Build history of the part. All positions in model axes, mm. Face numbers are marked on the shaded views. A direction names the side the tool comes from. Give positions to 0.01 mm unless a question says otherwise; leave off trailing zeros. Loops run counter-clockwise (first coordinate to the right, second up) from the corner with the lowest first, then second, coordinate; pieces in that order, holes last. Notation, with made-up numbers: (7.5, -12.5) -> (47.5, -12.5) arc R19 cw to (47.5, 6.5) -> close; hole circle Ø5 at (73.5, 86.5). An arc over 180 degrees is marked (long way). Answer as a JSON object with one key per item and string values. Group by question number.
Q1. Two-plate mould, pull along Y, no slides. Class the marked faces 3 and 4: pulls with the +Y half, pulls with the -Y half, needs draft (parallel to the pull), parting line crosses it, or undercut.
Q2. Band-saw the part on B-B, the plane y = 55.5. Write the cut outline in (x, z).
Q3. Drop flat-ended pins along their axis: pin 1 (4 mm diameter, centred on y = 151, z = 32.5, fed in from -X); pin 2 (3 mm diameter, centred on x = 140.5, z = 36.5, fed in from +Y); pin 3 (5 mm diameter, centred on x = 150, z = 96, fed in from +Y). Give the stop position or say it passes through.
Q4. Band-saw the part on A-A, the plane z = 17. Write the cut outline in (x, y), plus the area to 3 significant figures.
Q5. Tool access for the marked faces 1 and 2: list every direction of +Z, -Z, +X, -X, +Y, -Y with a clear straight run to the whole face (end or side of a thin tool).
Q6. Band-saw the part on C-C, the plane x = 102. Write the cut outline in (y, z).
Q7. Wall check: probe 1 along Y at (x, z) = (24.5, 78); probe 2 along Y at (x, z) = (134, 7); probe 3 along Z at (x, y) = (150, 1.5). Give the ranges that are in metal, low to high. Write a range as from..to.
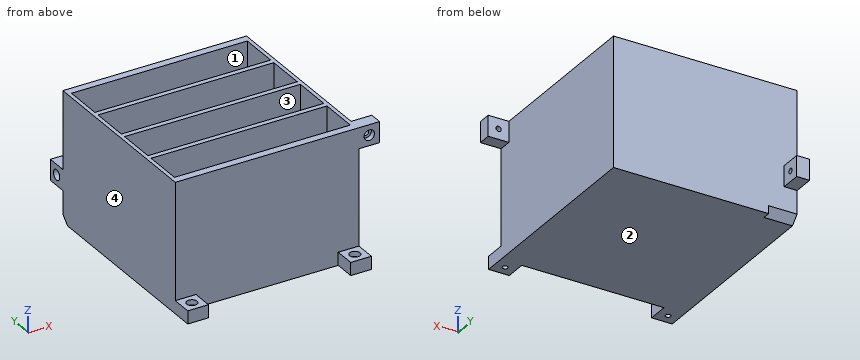
from build123d import *

# Parameters (mm, degrees)
SKETCH_W        = 142
SKETCH_H        = 144
PAD_DEPTH       = 100
SKETCH001_W     = 136
SKETCH001_H     = 30
POCKET_DEPTH    = 95
SKETCH002_W     = 10
SKETCH002_H     = 16
PAD001_DEPTH    = 16
SKETCH003_R     = 4
POCKET001_DEPTH = 4
SKETCH004_R     = 2
POCKET002_DEPTH = 6
SKETCH005_W     = 16
SKETCH005_H     = 10
PAD002_DEPTH    = 16
SKETCH006_R     = 4
POCKET003_DEPTH = 4
SKETCH007_R     = 2
POCKET004_DEPTH = 6
POCKET005_DEPTH = 22
SKETCH009_W     = 10
SKETCH009_H     = 16
PAD003_DEPTH    = 16
SKETCH010_R     = 4
POCKET006_DEPTH = 4
SKETCH011_R     = 2
POCKET007_DEPTH = 6


with BuildPart() as part:
    # Sketch → Pad (new body)
    with BuildSketch(Plane.XY):
        with Locations((71, 72)):
            Rectangle(SKETCH_W, SKETCH_H)
    extrude(amount=PAD_DEPTH)

    # Sketch001 (on Face6 of Pad) → Pocket (cut)
    with BuildSketch(Plane.XY.offset(100)):
        with Locations((71, 123)):
            Rectangle(SKETCH001_W, SKETCH001_H)
        with Locations((71, 89)):
            Rectangle(SKETCH001_W, SKETCH001_H)
        with Locations((71, 55)):
            Rectangle(SKETCH001_W, SKETCH001_H)
        with Locations((71, 21)):
            Rectangle(SKETCH001_W, SKETCH001_H)
    extrude(amount=-POCKET_DEPTH, mode=Mode.SUBTRACT)

    # Sketch002 (on Face1 of Pocket) → Pad001 (join)
    with BuildSketch(Plane(origin=(0, 144, 0), x_dir=(-1, 0, 0), z_dir=(0, 1, 0))):
        with Locations((-5, 32)):
            Rectangle(SKETCH002_W, SKETCH002_H)
    extrude(amount=PAD001_DEPTH)

    # Sketch003 (on Face10 of Pad001) → Pocket001 (cut)
    with BuildSketch(Plane(origin=(0, 0, 0), x_dir=(0, -1, 0), z_dir=(-1, 0, 0))):
        with Locations((-152, 32)):
            Circle(SKETCH003_R)
    extrude(amount=-POCKET001_DEPTH, mode=Mode.SUBTRACT)

    # Sketch004 (on Face33 of Pocket001) → Pocket002 (cut)
    with BuildSketch(Plane(origin=(4, 0, 0), x_dir=(0, -1, 0), z_dir=(-1, 0, 0))):
        with Locations((-152, 32)):
            Circle(SKETCH004_R)
    extrude(amount=-POCKET002_DEPTH, mode=Mode.SUBTRACT)

    # Sketch005 (on Face4 of Pocket002) → Pad002 (join)
    with BuildSketch(Plane.XZ):
        with Locations((8, 5)):
            Rectangle(SKETCH005_W, SKETCH005_H)
        with Locations((134, 5)):
            Rectangle(SKETCH005_W, SKETCH005_H)
    extrude(amount=PAD002_DEPTH)

    # Sketch006 (on Face38 of Pad002) → Pocket003 (cut)
    with BuildSketch(Plane.XY.offset(10)):
        with Locations((8, -8)):
            Circle(SKETCH006_R)
        with Locations((134, -8)):
            Circle(SKETCH006_R)
    extrude(amount=-POCKET003_DEPTH, mode=Mode.SUBTRACT)

    # Sketch007 (on Face48 of Pocket003) → Pocket004 (cut)
    with BuildSketch(Plane.XY.offset(6)):
        with Locations((8, -8)):
            Circle(SKETCH007_R)
        with Locations((134, -8)):
            Circle(SKETCH007_R)
    extrude(amount=-POCKET004_DEPTH, mode=Mode.SUBTRACT)

    # Sketch008 (on Face5 of Pocket004) → Pocket005 (cut)
    with BuildSketch(Plane(origin=(0, 0, 0), x_dir=(0, -1, 0), z_dir=(-1, 0, 0))):
        Polygon((-144, 6), (-144, 0), (-138, 0), align=None)
    extrude(amount=-POCKET005_DEPTH, mode=Mode.SUBTRACT)

    # Sketch009 (on Face3 of Pocket005) → Pad003 (join)
    with BuildSketch(Plane.YZ.offset(142)):
        with Locations((5, 92)):
            Rectangle(SKETCH009_W, SKETCH009_H)
    extrude(amount=PAD003_DEPTH)

    # Sketch010 (on Face42 of Pad003) → Pocket006 (cut)
    with BuildSketch(Plane.XZ):
        with Locations((150, 92)):
            Circle(SKETCH010_R)
    extrude(amount=-POCKET006_DEPTH, mode=Mode.SUBTRACT)

    # Sketch011 (on Face59 of Pocket006) → Pocket007 (cut)
    with BuildSketch(Plane.XZ.offset(-4)):
        with Locations((150, 92)):
            Circle(SKETCH011_R)
    extrude(amount=-POCKET007_DEPTH, mode=Mode.SUBTRACT)


solid = part.part
Worked answers:
{
 "1": {"face 3": "undercut", "face 4": "needs draft"},
 "2": {"outline": "(0, 0) -> (142, 0) -> (142, 100) -> (139, 100) -> (139, 5) -> (3, 5) -> (3, 100) -> (0, 100) -> close"},
 "3": {"pin 1": "x = 4", "pin 2": "y = 144", "pin 3": "y = 10"},
 "4": {"outline": "(0, 0) -> (142, 0) -> (142, 144) -> (0, 144) -> close; hole (3, 6) -> (139, 6) -> (139, 36) -> (3, 36) -> close; hole (3, 40) -> (139, 40) -> (139, 70) -> (3, 70) -> close; hole (3, 74) -> (139, 74) -> (139, 104) -> (3, 104) -> close; hole (3, 108) -> (139, 108) -> (139, 138) -> (3, 138) -> close", "area": "4,130 mm2"},
 "5": {"face 1": "+Z", "face 2": "-Z, +X, -X, +Y, -Y"},
 "6": {"outline": "(0, 0) -> (144, 0) -> (144, 100) -> (138, 100) -> (138, 5) -> (108, 5) -> (108, 100) -> (104, 100) -> (104, 5) -> (74, 5) -> (74, 100) -> (70, 100) -> (70, 5) -> (40, 5) -> (40, 100) -> (36, 100) -> (36, 5) -> (6, 5) -> (6, 100) -> (0, 100) -> close"},
 "7": {"probe 1": "0..6, 36..40, 70..74, 104..108, 138..144", "probe 2": "-16..-12, -4..6, 36..40, 70..74, 104..108, 138..144", "probe 3": "84..88, 96..100"}
}
